Autodesk Fusion 360 part; units mm, degrees
sketch "BaseSketch" plane through (0, 0, 0) normal (0, 0, 1) x (1, 0, 0)
  line L0 (-77, -32) -> (37, -32)
  arc A0 (37, -32) -> (37, 32) centre (37, 0) ccw
  line L1 (37, 32) -> (-77, 32)
  arc A1 (-77, 32) -> (-77, -32) centre (-77, 0) ccw
  line L2 (-77, 0) -> (37, 0) construction
  circle A2 centre (-77, 0) radius 11
  circle A3 centre (37, 0) radius 11
  line L3 (-77, 0) -> (-52, 0) construction
  line L4 (-52, 32) -> (10, 32) construction
  line L5 (10, 32) -> (10, -32)
  line L6 (10, -32) -> (-52, -32) construction
  line L7 (-52, -32) -> (-52, 32)
  line L8 (-39, -32) -> (-39, 19)
  line L9 (-39, 19) -> (-3, 19)
  line L10 (-3, 19) -> (-3, -32)
  dimension "d2" = 64
  dimension "d3" = 22
  dimension "d4" = 22
  dimension "d5" = 25
  dimension "d6" = 62
  dimension "d7" = 13
extrude "Extrude1" add sketch "BaseSketch" along normal blind 19 contours L0 L1 A1 L7 | L0 A0 L1 L5 makes body 1 at (15.3333, 0, 0) makes body 2 at (-66.8333, 24.5088, 0)
extrude "Extrude2" add sketch "BaseSketch" along normal blind 64 contours L0 L1 L5 L7 L8 L9 L10 bodies 1 2
extrude "Extrude3" add sketch "BaseSketch" along normal blind 19 contours L0 L8 L9 L10 bodies 1
sketch "TriangleSketch" plane through (0, 0, 0) normal (1, 0, 0) x (0, 1, 0)
  line L0 (32, 0) -> (19, 0)
  line L1 (19, 0) -> (-32, 0)
  line L2 (19, 0) -> (-32, 0)
  line L3 (-32, 0) -> (-32, 19)
  line L4 (-32, 19) -> (19, 19)
  line L5 (19, 19) -> (19, 0)
  line L6 (19, 19) -> (19, 64)
  line L7 (19, 64) -> (-32, 19)
  dimension "d14" = 13
  dimension "d15" = 51
  dimension "d16" = 19
extrude "Extrude4" add sketch "TriangleSketch" against normal blind 36 from surface at -3 contours L4 L6 L7 bodies 1
Build history of the part. All positions in model axes, mm. A direction names the side the tool comes from. Give positions to 0.01 mm unless a question says otherwise; leave off trailing zeros. Order: outer loops, then holes, each group sorted by start corner. A loop starts at its lowest first (then second) coordinate and runs counter-clockwise, first axis right, second up. Notation, with made-up numbers: M 74,10 L 92,10 A19 cw 92,33 Z; hole C 61,29 d10. An arc over 180 degrees is marked long. Use one line per item in the form item = value.
1) Saw through at D-D (y = 25.5). Give the cut face in (x, z), plus the area to 3 significant figures.
Calculated:
outline = M -96.33,0 L 56.33,0 L 56.33,19 L 10,19 L 10,64 L -52,64 L -52,19 L -96.33,19 Z
area = 5,690 mm2
2) Drop flat-ended pins along their axis: pin 1 (4 mm diameter, centred on y = 20.5, z = 14, fed in from +X); pin 2 (10 mm diameter, centred on x = 34, y = 13.5, fed in from +Z); pin 3 (1 mm diameter, centred on y = -15.5, z = 18, fed in from +X). Give the stop position or say it passes through.
Calculated:
pin_1 = 63.11
pin_2 = 19
pin_3 = 65.27
3) Saw through at A-A (x = 29). Give the cut face in (y, z).
Calculated:
outline = M -32,0 L -7.55,0 L -7.55,19 L -32,19 Z; M 7.55,0 L 32,0 L 32,19 L 7.55,19 Z
4) Tool access for faces 1 (the face through (-87, 8, 19)), 2 (the face through (-39, -18, 51)), 3 (the face through (46, 8, 19)): list every direction of +Z, -Z, +X, -X, +Y, -Y with a clear straight run to the whole face (end or side of a thin tool).
Calculated:
face_1 = +Z, -X, +Y, -Y
face_2 = +Z, -Y
face_3 = +Z, +X, +Y, -Y
5) Two-plate mould, pull along X, no slides. Class faces 4 (the face through (68.992, 0.704, 9.367)), 5 (the face through (-52, 0, 41)), 6 (the face through (-21, -32, 17)), 7 (the face through (-3, -17, 51)): released by +X, released by -X, zero draft, split by the parting line, or undercut.
Calculated:
face_4 = released by +X
face_5 = released by -X
face_6 = zero draft
face_7 = undercut
6) Probe probe 1 along X at (y, z) = (-19.5, 33); probe 2 along Y at (x, z) = (37, 6); probe 3 along Z at (x, y) = (17.5, 28). List the from-to ranges inside material, lowest first.
Calculated:
probe_1 = -52 to -39, -3 to 10
probe_2 = -32 to -11, 11 to 32
probe_3 = 0 to 19
7) Saw through at C-C (y = 2.5). Give the cut face in (x, z), plus the area to 3 significant figures.
Calculated:
outline = M -108.9,0 L -87.71,0 L -87.71,19 L -108.9,19 Z; M -66.29,0 L 26.29,0 L 26.29,19 L 10,19 L 10,64 L -3,64 L -3,49.44 L -39,49.44 L -39,64 L -52,64 L -52,19 L -66.29,19 Z; M 47.71,0 L 68.9,0 L 68.9,19 L 47.71,19 Z
area = 4,830 mm2
8) Saw through at B-B (z = 43). Give the cut face in (x, y), plus the area to 3 significant figures.
Calculated:
outline = M -52,-32 L -39,-32 L -39,-4.8 L -3,-4.8 L -3,-32 L 10,-32 L 10,32 L -52,32 Z
area = 2,990 mm2
